Input: dimensioned drawing with shaded views. Units: mm. Origin: part minimum x, y, z. A direction names the side the tool comes from. Give positions to 0.01 mm unless a question says otherwise; leave off trailing zeros. Order: outer loops, then holes, each group sorted by start corner. A loop starts at its lowest first (then second) coordinate and runs counter-clockwise, first axis right, second up. Notation, with made-up numbers: (17.5, 27) -> (43.5, 27) arc R23 cw to (43.5, 45) -> close; hole circle Ø7 at (21, 60). An arc over 180 degrees is marked (long way). Use CSV: the item, a comma, the result in double quotes.
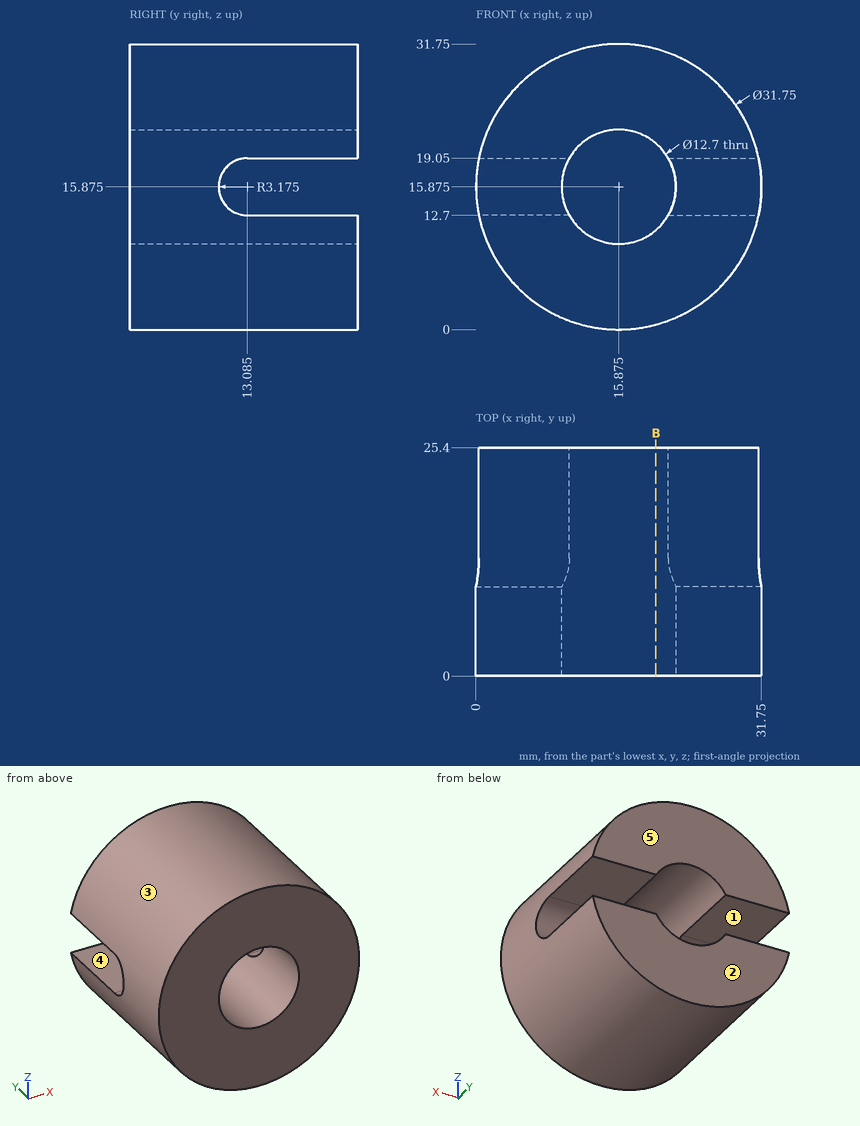
1. Mould query, pull axis Z, two halves, no side actions, for the marked faces 3, 4 and 5. Classes: released by +Z, released by -Z, zero draft, split by the parting line, or undercut.
Answer below:
face 3,"split by the parting line"
face 4,"undercut"
face 5,"zero draft"
2. Access query for the marked faces 1 and 2. Directions: +Z, -Z, +X, -X, +Y, -Y. A direction counts if a zero-diameter tool reaches every point of the face in a straight line with its end or side. Return the directions, or none.
Answer below:
face 1,"+X, -X, +Y"
face 2,"+Z, -Z, +X, -X, +Y"
3. Section query B-B on x = 20. Return loops of the section in (y, z) (1 decimal).
Answer below:
outline,"(0, 0.5) -> (25.4, 0.5) -> (25.4, 11) -> (0, 11) -> close; (0, 20.7) -> (25.4, 20.7) -> (25.4, 31.2) -> (0, 31.2) -> close"
4. Ray query, line 1 along Z through (x, y) = (15.5, 24) (1 decimal); line 2 along X through (y, z) = (18.5, 21.5) (1 decimal); line 3 along Z through (x, y) = (14, 7.75). Return the intervals inside material, ascending.
Answer below:
line 1,"z = 0 to 9.5, 22.2 to 31.7"
line 2,"x = 1 to 12.9, 18.8 to 30.7"
line 3,"z = 0.11 to 9.81, 21.94 to 31.64"
5. Pin query (flat end, axial travel): P1, Ø3, axis at x = 22.5, y = 9.5, coming from the +Z side; P2, Ø11.5, axis at x = 15.875, z = 15.875, coming from the -Y side; P3, Ø6, axis at y = 20.5, z = 16.5, coming from the +X side; P4, Ø11, axis at x = 6.5, y = 20, coming from the +Z side. Return the tip coordinate at first contact, or that it passes through.
Answer below:
P1,"stops at z = 30.9"
P2,"passes through"
P3,"stops at x = 31.43"
P4,"stops at z = 31.27"
